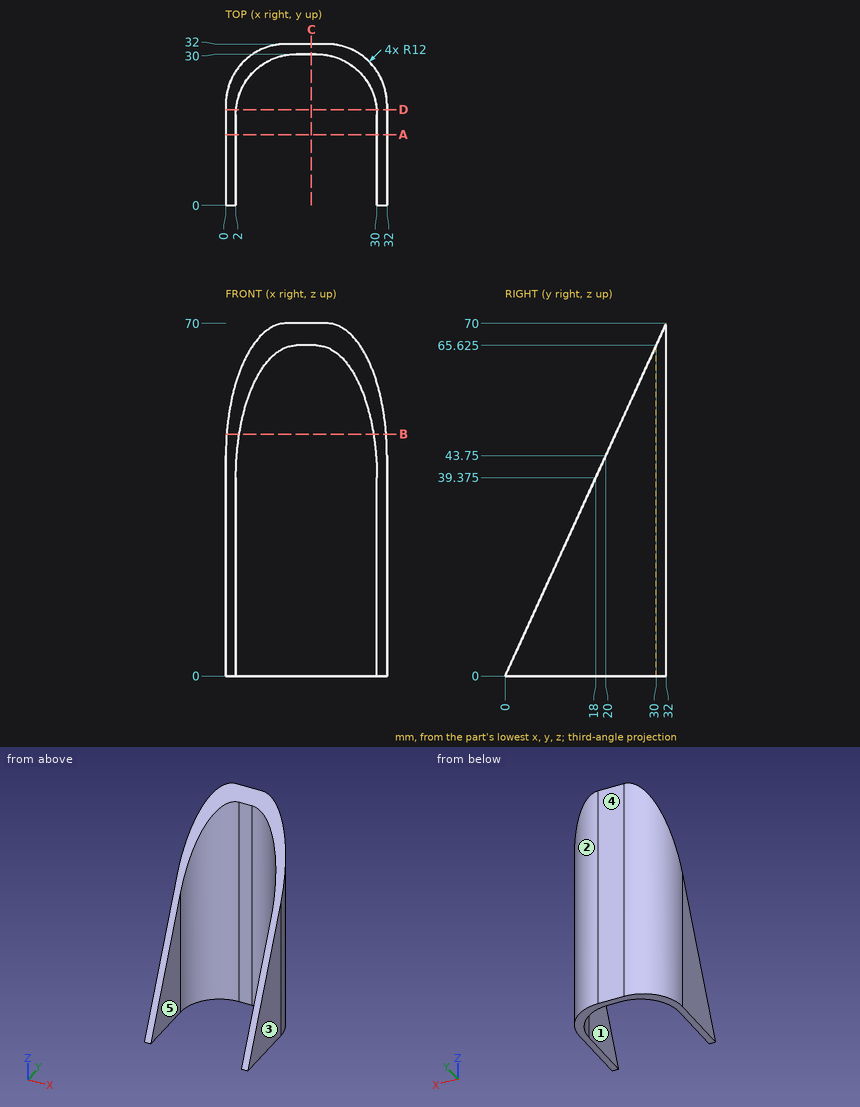
Geometry check sheet. Reference: drawing and pictorial views, mm from the part's lowest x, y, z. A direction names the side the tool comes from. Give positions to 0.01 mm unless a question says otherwise; leave off trailing zeros. Write each loop counter-clockwise with the first axis right and the second up, starting at its lowest first coordinate (ties: lowest second). Pieces come first, ordered by that corner, then holes. Notation, with made-up numbers: (-4.5, 77) - (7.5, 77) arc R38 cw to (7.5, 116) - close; hole circle Ø10 at (20, -10.75). An arc over 180 degrees is marked (long way). Use a Markdown table: item, result.
Q1. Draft check along X on the marked faces 3, 4 and 5. Enter one of: pulls with the +X half, pulls with the -X half, needs draft (parallel to the pull), parting line crosses it, or undercut.
Computed:
| item | result |
|---|---|
| face 3 | pulls with the +X half |
| face 4 | needs draft |
| face 5 | undercut |
Q2. Thickness scan on L1, parallel to X at y = 17, z = 17.5; L2, parallel to Y at x = 15.5, z = 44; L3, parallel to X at y = 25, z = 52.5. Record the ranges inside material, lowest first. Write a range as [from, to].
Computed:
| item | result |
|---|---|
| L1 | x = [0, 2], [30, 32] |
| L2 | y = [30, 32] |
| L3 | x = [1.09, 4.25], [27.75, 30.91] |
Q3. Go/stop test with flat-tipped pins: P1, Ø12, axis at x = 16.5, y = 25.5, coming from the +Z side; P2, Ø10, axis at y = 25.5, z = 46, coming from the +X side; P3, Ø10, axis at x = 11.5, z = 60.5, coming from the -Y side. Record where each tip stops, or that it passes through.
Computed:
| item | result |
|---|---|
| P1 | stops at z = 68.91 |
| P2 | stops at x = 31.99 |
| P3 | stops at y = 27.39 |
Q4. Set-up check for the marked faces 1 and 2: record each of +Z, -Z, +X, -X, +Y, -Y from which the full face is reachable in a straight line by a thin tool's end or side.
Computed:
| item | result |
|---|---|
| face 1 | +Z, -Z, -Y |
| face 2 | +Z, -Z, +X, +Y |
Q5. Section check B-B, the plane z = 48. Enter the section's corners in (x, y).
Computed:
| item | result |
|---|---|
| outline | (0.16, 21.94) - (2.67, 21.94) arc R12 cw to (14, 30) - (18, 30) arc R12 cw to (29.33, 21.94) - (31.84, 21.94) arc R12 ccw to (20, 32) - (12, 32) arc R12 ccw to start |
Q6. Section check D-D, the plane y = 19. Enter the section's corners in (x, z).
Computed:
| item | result |
|---|---|
| outline | (0, 0) - (2.04, 0) - (2.04, 41.56) - (0, 41.56) - close; (29.96, 0) - (32, 0) - (32, 41.56) - (29.96, 41.56) - close |
Q7. Section check A-A, the plane y = 14. Enter the section's corners in (x, z) (3 decimals).
Computed:
| item | result |
|---|---|
| outline | (0, 0) - (2, 0) - (2, 30.625) - (0, 30.625) - close; (30, 0) - (32, 0) - (32, 30.625) - (30, 30.625) - close |
Q8. Section check C-C, the plane x = 17. Enter the section's corners in (y, z) (3 decimals).
Computed:
| item | result |
|---|---|
| outline | (30, 0) - (32, 0) - (32, 70) - (30, 65.625) - close |
